from build123d import *

# Parameters (mm, degrees)
SKETCH1_W           = 70
SKETCH1_H           = 70
SKETCH1_R           = 2.5
SKETCH1_W_2         = 22
SKETCH1_H_2         = 42
BOSS_EXTRUDE1_DEPTH = 12.5
SKETCH3_W           = 10.391499035
SKETCH3_H           = 15
SKETCH3_W_2         = 5.21700193
BOSS_EXTRUDE2_DEPTH = 15
SKETCH8_W           = 70
SKETCH8_H           = 42.5
BOSS_EXTRUDE5_DEPTH = 5
SKETCH12_W          = 70
SKETCH12_H          = 5
BOSS_EXTRUDE6_DEPTH = 30


with BuildPart() as part:
    # Sketch1 → Boss-Extrude1 (new body)
    with BuildSketch(Plane(origin=(0, 0, 0), x_dir=(1, 0, 0), z_dir=(0, 1, 0))):
        Rectangle(SKETCH1_W, SKETCH1_H)
        with Locations(Location((-18.608500965, 24, 0), (0, 0, 270))):
            Circle(SKETCH1_R, mode=Mode.SUBTRACT)
        with Locations(Location((-8.608500965, 24, 0), (0, 0, 270))):
            Circle(SKETCH1_R, mode=Mode.SUBTRACT)
        with Locations(Location((-8.608500965, -24, 0), (0, 0, 90))):
            Circle(SKETCH1_R, mode=Mode.SUBTRACT)
        with Locations(Location((-18.608500965, -24, 0), (0, 0, 90))):
            Circle(SKETCH1_R, mode=Mode.SUBTRACT)
        with Locations(Location((8.608500965, -24, 0), (0, 0, 270))):
            Circle(SKETCH1_R, mode=Mode.SUBTRACT)
        with Locations(Location((18.608500965, -24, 0), (0, 0, 270))):
            Circle(SKETCH1_R, mode=Mode.SUBTRACT)
        with Locations(Location((8.608500965, 24, 0), (0, 0, 90))):
            Circle(SKETCH1_R, mode=Mode.SUBTRACT)
        with Locations(Location((18.608500965, 24, 0), (0, 0, 90))):
            Circle(SKETCH1_R, mode=Mode.SUBTRACT)
        with Locations((-13.608500965, 0)):
            Rectangle(SKETCH1_W_2, SKETCH1_H_2, mode=Mode.SUBTRACT)
        with Locations((13.608500965, 0)):
            Rectangle(SKETCH1_W_2, SKETCH1_H_2, mode=Mode.SUBTRACT)
    extrude(amount=BOSS_EXTRUDE1_DEPTH)

    # Sketch3 → Boss-Extrude2 (add)
    with BuildSketch(Plane.XZ):
        with Locations((-29.804250483, 0)):
            Rectangle(SKETCH3_W, SKETCH3_H)
        Rectangle(SKETCH3_W_2, SKETCH3_H)
        with Locations((29.804250483, 0)):
            Rectangle(SKETCH3_W, SKETCH3_H)
    extrude(amount=BOSS_EXTRUDE2_DEPTH)

    # Sketch8 → Boss-Extrude5 (add)
    with BuildSketch(Plane.XZ.offset(15)):
        Rectangle(SKETCH8_W, SKETCH8_H)
    extrude(amount=BOSS_EXTRUDE5_DEPTH)

    # Sketch12 → Boss-Extrude6 (add)
    with BuildSketch(Plane.XY.offset(21.25)):
        with Locations((0, -17.5)):
            Rectangle(SKETCH12_W, SKETCH12_H)
    extrude(amount=BOSS_EXTRUDE6_DEPTH)


solid = part.part
Can you work these out from the model? Positions are in its coordinate system, mm. A direction names the side the tool comes from. Give positions to 0.01 mm unless a question says otherwise; leave off trailing zeros. Loops run counter-clockwise (first coordinate to the right, second up) from the corner with the lowest first, then second, coordinate; pieces in that order, holes last. Notation, with made-up numbers: (-35.5, -8) - (-15.5, -8) arc R19 cw to (-15.5, 19) - close; hole circle Ø3 at (31, 16.5). An arc over 180 degrees is marked (long way). Answer as a JSON object with one key per item and string values.
Q1. Which directions (+Z, -Z, +X, -X, +Y, -Y) give clear straight access to the entire face, cutting with the end or side of a thin tool? Please do faces 5 (the flat face through (0, 0, 24)), 6 (the cylindrical face through (-17.087, 6.162, 25.984)), 7 (the flat face through (0, 0, -24)).
Geometry says:
{"face 5": "+Z, +X, -X", "face 6": "+Y", "face 7": "-Z, +X, -X"}
Q2. If I drill on L1, parallel to X at y = 3.25, z = -24; L2, parallel to X at y = 5.5, z = 2; L3, parallel to Y at x = -11.5, z = 33, over which ranges is the centre line in solid material (lowest first)?
Geometry says:
{"L1": "-35 to -21.11, -16.11 to -11.11, -6.11 to 6.11, 11.11 to 16.11, 21.11 to 35", "L2": "-35 to -24.61, -2.61 to 2.61, 24.61 to 35", "L3": "-20 to -15, 0 to 12.5"}
Q3. Will these pins go through, and if not, where does the flat tip stop? P1, Ø1.5, axis at x = 11, y = -17, coming from the -Z side; P2, Ø4.5, axis at x = -18.61, z = 24, coming from the +Y side; P3, Ø1.6, axis at x = 1, y = -10, coming from the +Z side.
Geometry says:
{"P1": "z = -21.25", "P2": "y = -15", "P3": "z = 7.5"}
Q4. Imagine slicing it at D-D on z = 34. Write out the boundary of the cut face in (x, y).
Geometry says:
{"outline": "(-35, -20) - (35, -20) - (35, -15) - (-35, -15) - close; (-35, 0) - (35, 0) - (35, 12.5) - (-35, 12.5) - close"}
Q5. If we mould it in two halves opening along Y, with no side actions, what happens to faces 1 (the cylindrical face through (-16.919, 6.162, -25.843)), 2 (the flat face through (0, 12.5, 0)), 3 (the flat face through (-30, -7, 7.5)), 4 (the flat face through (0, -20, 14))? For each: pulls with the +Y half, pulls with the -Y half, needs draft (parallel to the pull), parting line crosses it, or undercut.
Geometry says:
{"face 1": "needs draft", "face 2": "pulls with the +Y half", "face 3": "undercut", "face 4": "pulls with the -Y half"}
Q6. Imagine slicing it at B-B on z = -24. Write out the boundary of the cut face in (x, y), plus the area to 3 significant figures.
Geometry says:
{"outline": "(-35, 0) - (-21.11, 0) - (-21.11, 12.5) - (-35, 12.5) - close; (-16.11, 0) - (-11.11, 0) - (-11.11, 12.5) - (-16.11, 12.5) - close; (-6.11, 0) - (6.11, 0) - (6.11, 12.5) - (-6.11, 12.5) - close; (11.11, 0) - (16.11, 0) - (16.11, 12.5) - (11.11, 12.5) - close; (21.11, 0) - (35, 0) - (35, 12.5) - (21.11, 12.5) - close", "area": "625 mm²"}
Q7. Imagine slicing it at C-C on z = 24. Write out the boundary of the cut face in (x, y).
Geometry says:
{"outline": "(-35, -20) - (35, -20) - (35, -15) - (-35, -15) - close; (-35, 0) - (-21.11, 0) - (-21.11, 12.5) - (-35, 12.5) - close; (-16.11, 0) - (-11.11, 0) - (-11.11, 12.5) - (-16.11, 12.5) - close; (-6.11, 0) - (6.11, 0) - (6.11, 12.5) - (-6.11, 12.5) - close; (11.11, 0) - (16.11, 0) - (16.11, 12.5) - (11.11, 12.5) - close; (21.11, 0) - (35, 0) - (35, 12.5) - (21.11, 12.5) - close"}
Q8. Imagine slicing it at A-A on y = -10.5. Write out the boundary of the cut face in (x, z), plus the area to 3 significant figures.
Geometry says:
{"outline": "(-35, -7.5) - (-24.61, -7.5) - (-24.61, 7.5) - (-35, 7.5) - close; (-2.61, -7.5) - (2.61, -7.5) - (2.61, 7.5) - (-2.61, 7.5) - close; (24.61, -7.5) - (35, -7.5) - (35, 7.5) - (24.61, 7.5) - close", "area": "390 mm²"}
